Part model, mm, in its own coordinate system. A direction names the side the tool comes from. Give positions to 0.01 mm unless a question says otherwise; leave off trailing zeros. Order: outer loops, then holes, each group sorted by start corner. A loop starts at its lowest first (then second) coordinate and runs counter-clockwise, first axis right, second up. Notation, with made-up numbers: (76.25, 72.5) - (85.25, 72.5) arc R17 ccw to (85.25, 90.5) - close; hole circle Ø7 at (80, 23.25). An arc over 180 degrees is marked (long way). One line per item, written item: value.
```python
from build123d import *

# Parameters (mm, degrees)
F3_DEPTH = 12.75
F4_R     = 6
F5_DEPTH = 15


with BuildPart() as f1:
    # F0 (on Front) → F1 (revolve)
    with BuildSketch(Plane.XZ):
        Polygon((12, 286.387794), (0, 286.387794), (0, -56.612206), (10, -56.612206), (10, -36.612206), (8, -36.612206), (8, 263.387794), (12, 263.387794), align=None)
    revolve(axis=Axis((0, 0, 114.887794), (0, 0, 1)))

    # F2 (on face) → F3 (cut)
    with BuildSketch(Plane(origin=(0, 0, -56.612206), x_dir=(1, 0, 0), z_dir=(0, 0, -1))):
        with BuildLine():
            Line((3, 9.539392), (3, 0))
            Line((3, 0), (3, -9.539392))
            ThreePointArc((3, -9.539392), (8.062258, -5.91608), (10, 0))
            ThreePointArc((10, 0), (8.062258, 5.91608), (3, 9.539392))
        make_face()
        with BuildLine():
            Line((-3, -9.539392), (-3, 0))
            Line((-3, 0), (-3, 9.539392))
            ThreePointArc((-3, 9.539392), (-10, 0), (-3, -9.539392))
        make_face()
    extrude(amount=-F3_DEPTH, mode=Mode.SUBTRACT)

    # F4 (on face) → F5 (cut)
    with BuildSketch(Plane.XY.offset(286.387794)):
        Circle(F4_R)
    extrude(amount=-F5_DEPTH, mode=Mode.SUBTRACT)


solid = f1.part
```
1) Wall check: line 1 along Y through (x, z) = (0, 274.75); line 2 along Z through (x, y) = (-2.25, 8.75); line 3 along Z through (x, y) = (9.5, 4.5). Give the ranges that are in metal, low to high. Write a range as [from, to].
Answer:
line 1: y = [-12, -6], [6, 12]
line 2: z = [-56.61, -36.61], [263.39, 286.39]
line 3: z = [263.39, 286.39]
2) Drop flat-ended pins along their axis: P1, Ø9.5, axis at x = 0, y = 0, coming from the +Z side; P2, Ø12, axis at x = 9, z = 31.5, coming from the -Y side; P3, Ø14, axis at y = -3.5, z = -48.5, coming from the +X side. Give the stop position or say it passes through.
Answer:
P1: stops at z = 271.39
P2: stops at y = -7.42
P3: stops at x = 10
3) Two-plate mould, pull along Z, no slides. Class faces 6 (the face through (-2, -8, 263.388)), 7 (the face through (3, 0, -50)), 8 (the face through (0, 0, 271.388)), 9 (the face through (6, 0, -43.862)): pulls with the +Z half, pulls with the -Z half, needs draft (parallel to the pull), parting line crosses it, or undercut.
Answer:
face 6: undercut
face 7: needs draft
face 8: pulls with the +Z half
face 9: pulls with the -Z half
4) Slice it at B-B on y = 0. Write the cut outline in (x, z), then the cut area to 3 significant figures.
Answer:
outline: (-12, 263.39) - (-8, 263.39) - (-8, -36.61) - (-10, -36.61) - (-10, -43.86) - (-3, -43.86) - (-3, -56.61) - (3, -56.61) - (3, -43.86) - (10, -43.86) - (10, -36.61) - (8, -36.61) - (8, 263.39) - (12, 263.39) - (12, 286.39) - (6, 286.39) - (6, 271.39) - (-6, 271.39) - (-6, 286.39) - (-12, 286.39) - close
area: 5,390 mm2
5) Slice it at A-A on x = 0. Write the cut outline in (y, z).
Answer:
outline: (-12, 263.39) - (-8, 263.39) - (-8, -36.61) - (-10, -36.61) - (-10, -56.61) - (10, -56.61) - (10, -36.61) - (8, -36.61) - (8, 263.39) - (12, 263.39) - (12, 286.39) - (6, 286.39) - (6, 271.39) - (-6, 271.39) - (-6, 286.39) - (-12, 286.39) - close
6) Slice it at C-C on z = 139.5. Write the cut outline in (x, y).
Answer:
outline: circle Ø16 at (0, 0)
7) Which spindle directions (+Z, -Z, +X, -X, +Y, -Y) get a long thin tool onto all of the face, cutting with end or side? Do faces 1 (the face through (-1.73, -7.81, 115.49)), 2 (the face through (0, 0, -56.612)), 3 (the face through (-6, 0, 279)), 4 (the face through (-6, 0, -43.862)), 5 (the face through (-10, 0, -42)). Say none if no direction does.
Answer:
face 1: none
face 2: -Z, +X, -X, +Y, -Y
face 3: +Z
face 4: -Z, -X, +Y, -Y
face 5: -Z
